Could you check a few things on this drawing? It's one solid part, dimensions in mm from its lowest x, y, z. A direction names the side the tool comes from. Give positions to 0.01 mm unless a question says otherwise; leave off trailing zeros. Order: outer loops, then holes, each group sorted by start corner. A loop starts at its lowest first (then second) coordinate and runs counter-clockwise, first axis right, second up. Notation, with made-up numbers: (47, 46.5) - (85, 46.5) arc R20 ccw to (85, 85.5) - close; hole circle Ø5 at (59.5, 79.25). An arc over 180 degrees is marked (long way). Put each result on its own line as item: value.
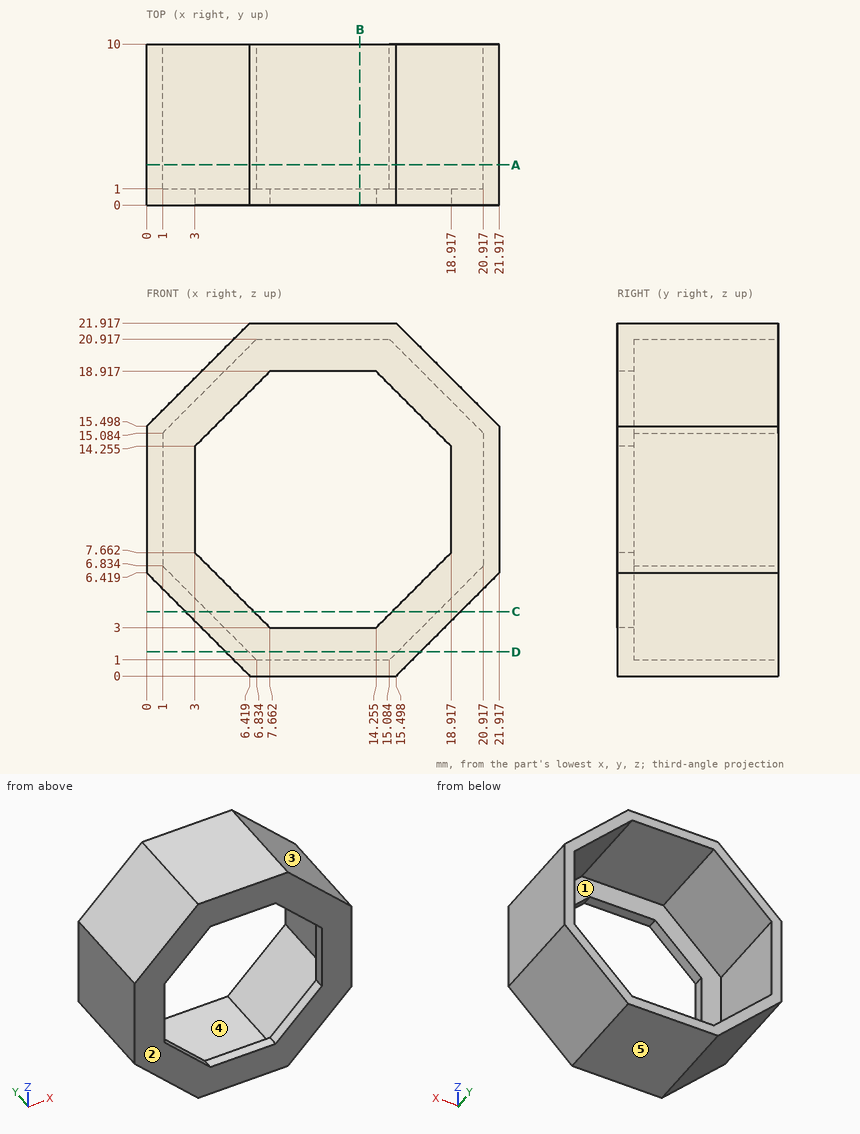
1) I'm going to push a flat-ended pin straight in: pin 1 (2 mm diameter, centred on y = 1.5, z = 18, fed in from -X). Where does the tip first touch, or does it pass through?
Filled in:
pin 1: stops at x = 1.5
2) Suppose I cut it at D-D, the plane z = 1.5. List the corners of the cut face in (x, y) for me.
Filled in:
outline: (4.92, 0) - (17, 0) - (17, 10) - (15.58, 10) - (15.58, 1) - (6.33, 1) - (6.33, 10) - (4.92, 10) - close
3) If I drill on line 1 (X direction, y = 8, z = 11.25); line 2 (Y direction, x = 4, z = 17), over which ranges is the centre line in solid material (lowest first)? Write a range as [from, to].
Filled in:
line 1: x = [0, 1], [20.92, 21.92]
line 2: y = [0, 1]
4) Which directions (+Z, -Z, +X, -X, +Y, -Y) give clear straight access to the entire face, cutting with the end or side of a thin tool? Please do the marked faces 4 and 5.
Filled in:
face 4: +Y
face 5: -Z, +X, -X, +Y, -Y
5) Suppose I cut it at B-B, the plane x = 13.25. List the corners of the cut face in (y, z) for me, and give its area (3 significant figures).
Filled in:
outline: (0, 0) - (10, 0) - (10, 1) - (1, 1) - (1, 3) - (0, 3) - close; (0, 18.92) - (1, 18.92) - (1, 20.92) - (10, 20.92) - (10, 21.92) - (0, 21.92) - close
area: 24.0 mm^2
6) Suppose I cut it at C-C, the plane z = 4. List the corners of the cut face in (x, y) for me (1 decimal).
Filled in:
outline: (2.4, 0) - (6.7, 0) - (6.7, 1) - (3.8, 1) - (3.8, 10) - (2.4, 10) - close; (15.3, 0) - (19.5, 0) - (19.5, 10) - (18.1, 10) - (18.1, 1) - (15.3, 1) - close
7) Suppose I cut it at A-A, the plane y = 2.5. List the corners of the cut face in (x, z) for me.
Filled in:
outline: (0, 6.42) - (6.42, 0) - (15.5, 0) - (21.92, 6.42) - (21.92, 15.5) - (15.5, 21.92) - (6.42, 21.92) - (0, 15.5) - close; hole (1, 6.83) - (6.83, 1) - (15.08, 1) - (20.92, 6.83) - (20.92, 15.08) - (15.08, 20.92) - (6.83, 20.92) - (1, 15.08) - close
8) We'd pull the mould along Z, two halves only. Please class the marked faces 1, 2 and 3: pulls with the +Z half, pulls with the -Z half, needs draft (parallel to the pull), parting line crosses it, or undercut.
Filled in:
face 1: undercut
face 2: needs draft
face 3: pulls with the +Z half
